Could you check a few things on this drawing? It's one solid part, dimensions in mm from its lowest x, y, z. Give positions to 0.01 mm unless a question says otherwise; leave off trailing zeros. Loops run counter-clockwise (first coordinate to the right, second up) from the corner with the lowest first, then second, coordinate; pieces in that order, holes last. Notation, with made-up numbers: (-30, 32.5) -> (28, 32.5) arc R24 ccw to (28, 46.5) -> close; hole circle Ø1 at (-13, 21). An arc over 180 degrees is marked (long way). Use CSV: the item, a comma, the result in double quotes.
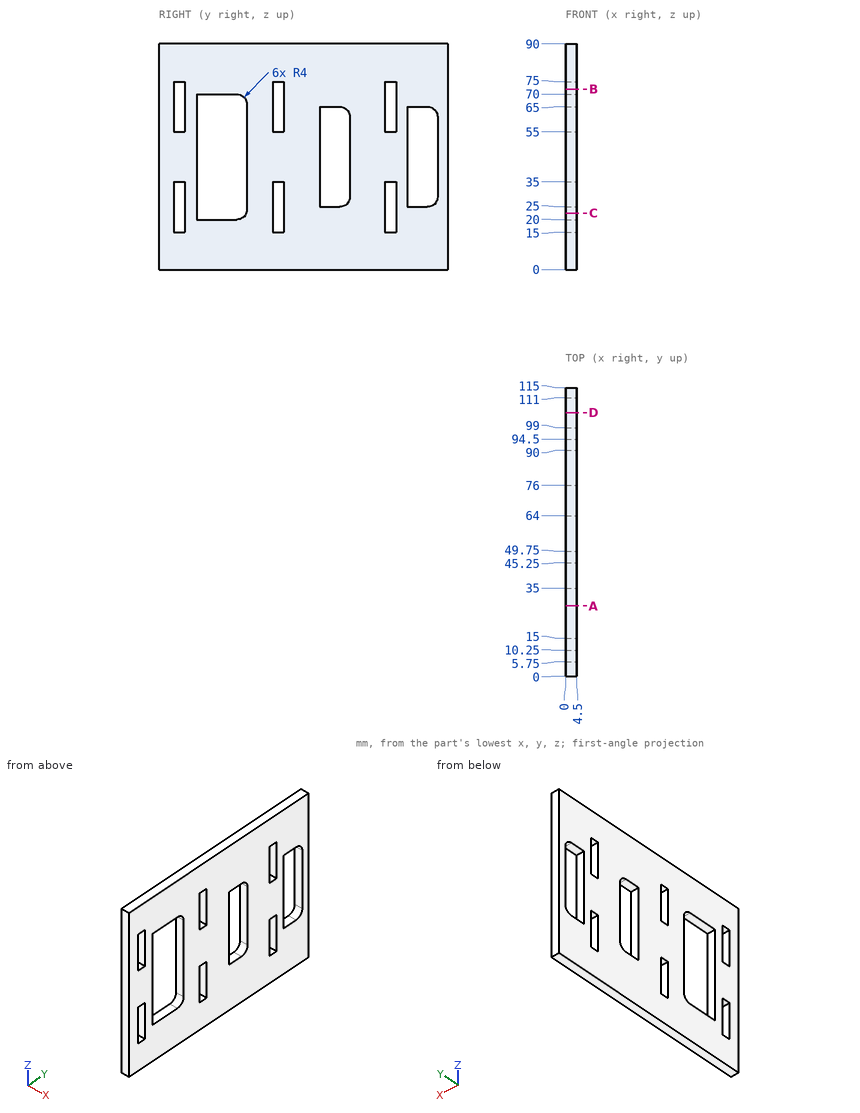
(1) If we section it at A-A, the plane y = 28: Write out the boundary of the cut face in (x, z).
Answer sheet:
outline,"(0, 0) -> (4.5, 0) -> (4.5, 20) -> (0, 20) -> close; (0, 70) -> (4.5, 70) -> (4.5, 90) -> (0, 90) -> close"
(2) If we section it at B-B, the plane z = 72: Write out the boundary of the cut face in (x, y).
Answer sheet:
outline,"(0, 0) -> (4.5, 0) -> (4.5, 5.75) -> (0, 5.75) -> close; (0, 10.25) -> (4.5, 10.25) -> (4.5, 45.25) -> (0, 45.25) -> close; (0, 49.75) -> (4.5, 49.75) -> (4.5, 90) -> (0, 90) -> close; (0, 94.5) -> (4.5, 94.5) -> (4.5, 115) -> (0, 115) -> close"
(3) If we section it at D-D, the plane y = 105: Write out the boundary of the cut face in (x, z), then the cut area to 3 significant figures.
Answer sheet:
outline,"(0, 0) -> (4.5, 0) -> (4.5, 25) -> (0, 25) -> close; (0, 65) -> (4.5, 65) -> (4.5, 90) -> (0, 90) -> close"
area,"225 mm2"
(4) If I drill on L1, parallel to Z at x = 2.1, y = 8; L2, parallel to Y at x = 1.8, z = 47; L3, parallel to Z at x = 1.2, y = 30, over which ranges is the centre line in solid material (lowest first)? Write a range as from..to.
Answer sheet:
L1,"z = 0..15, 35..55, 75..90"
L2,"y = 0..15, 35..64, 76..99, 111..115"
L3,"z = 0..20, 70..90"
(5) If we section it at C-C, the plane z = 22.5: Write out the boundary of the cut face in (x, y), then the cut area to 3 significant figures.
Answer sheet:
outline,"(0, 0) -> (4.5, 0) -> (4.5, 5.75) -> (0, 5.75) -> close; (0, 10.25) -> (4.5, 10.25) -> (4.5, 15) -> (0, 15) -> close; (0, 34.71) -> (4.5, 34.71) -> (4.5, 45.25) -> (0, 45.25) -> close; (0, 49.75) -> (4.5, 49.75) -> (4.5, 90) -> (0, 90) -> close; (0, 94.5) -> (4.5, 94.5) -> (4.5, 115) -> (0, 115) -> close"
area,"368 mm2"
(6) Will these pins go through, and if not, where does the flat tip stop? pin 1 Ø1.3 at (x, y) = (2.5, 7.5) entering from -Z; pin 2 Ø2 at (y, z) = (33.5, 28.5) entering from -X.
Answer sheet:
pin 1,"stops at z = 0"
pin 2,"passes through"
